from build123d import *

# Parameters (mm, degrees)
SKETCH1_R           = 2
SKETCH1_R_2         = 2.25
SKETCH1_R_3         = 16
SKETCH1_R_4         = 5.5
SKETCH1_R_5         = 1.75
SKETCH1_R_6         = 8.75
BOSS_EXTRUDE1_DEPTH = 3
SKETCH2_R           = 1.5
CUT_EXTRUDE1_DEPTH  = 190.515777006


with BuildPart() as part:
    # Sketch1 → Boss-Extrude1 (new body)
    with BuildSketch(Plane.XY):
        with BuildLine():
            ThreePointArc((-111.886028634, 49.480245878), (-128.824449864, 42.592956949), (-134.705774542, 25.279526249))
            ThreePointArc((-134.705774542, 25.279526249), (-136.343375771, 16.802270376), (-142.382746132, 10.632050724))
            ThreePointArc((-142.382746132, 10.632050724), (-155.099864059, -8.058287742), (-147.542861296, -29.364285714))
            ThreePointArc((-147.542861296, -29.364285714), (-143.125485566, -32.280163581), (-137.970351553, -33.480224156))
            ThreePointArc((-137.970351553, -33.480224156), (-126.431132561, -39.888203569), (-124.422839539, -52.93360637))
            ThreePointArc((-124.422839539, -52.93360637), (-124.888175134, -64.31939994), (-119.594822483, -74.410646153))
            Line((-119.594822483, -74.410646153), (-92.540517723, -103.740413224))
            ThreePointArc((-92.540517723, -103.740413224), (-82.119700521, -108.557935129), (-71.344567605, -104.595807028))
            Line((-71.344567605, -104.595807028), (-31.441449774, -67.788453323))
            ThreePointArc((-31.441449774, -67.788453323), (-26.802171393, -64.493076397), (-21.481893225, -62.473904985))
            Line((-21.481893225, -62.473904985), (87.599861039, -36.324111832))
            ThreePointArc((87.599861039, -36.324111832), (89.628937626, -35.308169791), (91, -33.5))
            ThreePointArc((91, -33.5), (97.203558128, 3.661751943), (84.51565505, 39.137054004))
            ThreePointArc((84.51565505, 39.137054004), (82.813644384, 40.69192784), (80.594954641, 41.317938046))
            Line((80.594954641, 41.317938046), (-111.886028634, 49.480245878))
        make_face()
        with Locations((-81.514845762, -93.570135067)):
            Circle(SKETCH1_R, mode=Mode.SUBTRACT)
        with Locations((-138.3, -22.75)):
            Circle(SKETCH1_R, mode=Mode.SUBTRACT)
        with Locations((-138.3, -5.25)):
            Circle(SKETCH1_R, mode=Mode.SUBTRACT)
        with Locations((-68.3, -21.5)):
            Circle(SKETCH1_R_2, mode=Mode.SUBTRACT)
        with Locations((-74.1, 1.7)):
            Circle(SKETCH1_R_2, mode=Mode.SUBTRACT)
        with Locations((-112.818118288, 27.5)):
            Circle(SKETCH1_R_3, mode=Mode.SUBTRACT)
        with Locations((-65.4, 20.2)):
            Circle(SKETCH1_R_2, mode=Mode.SUBTRACT)
        with Locations((18.5, -8.7)):
            Circle(SKETCH1_R_2, mode=Mode.SUBTRACT)
        with Locations((8.1, 8.2)):
            Circle(SKETCH1_R_2, mode=Mode.SUBTRACT)
        with Locations((75.9, -21.8)):
            Circle(SKETCH1_R_2, mode=Mode.SUBTRACT)
        with Locations((40.017782272, 0)):
            Circle(SKETCH1_R_4, mode=Mode.SUBTRACT)
        with Locations((78, -0.1)):
            Circle(SKETCH1_R_2, mode=Mode.SUBTRACT)
        with Locations((73, 22.4)):
            Circle(SKETCH1_R_2, mode=Mode.SUBTRACT)
        with Locations((-90.498978695, -58.098516388)):
            Circle(SKETCH1_R_5, mode=Mode.SUBTRACT)
        with Locations((-102.02811514, -72.419096433)):
            Circle(SKETCH1_R_5, mode=Mode.SUBTRACT)
        with Locations((-116.348695186, -60.889959988)):
            Circle(SKETCH1_R_5, mode=Mode.SUBTRACT)
        with Locations((-103.42383694, -59.494238188)):
            Circle(SKETCH1_R_6, mode=Mode.SUBTRACT)
        with Locations((-104.819558741, -46.569379943)):
            Circle(SKETCH1_R_5, mode=Mode.SUBTRACT)
    extrude(amount=BOSS_EXTRUDE1_DEPTH)

    # Sketch2 → Cut-Extrude1 (cut, through all)
    with BuildSketch(Plane.XY.offset(3)):
        with Locations((80.467851506, 38.32063179)):
            Circle(SKETCH2_R)
        with Locations((0.467851506, 41.713094856)):
            Circle(SKETCH2_R)
        with Locations((-79.532148494, 45.105557921)):
            Circle(SKETCH2_R)
        with Locations((86.900496491, -33.406768995)):
            Circle(SKETCH2_R)
        with Locations((9.034770729, -52.073251177)):
            Circle(SKETCH2_R)
        with Locations((-152.133709173, -14)):
            Circle(SKETCH2_R)
        with Locations((-68.830955034, -70.73973336)):
            Circle(SKETCH2_R)
    extrude(amount=-CUT_EXTRUDE1_DEPTH, mode=Mode.SUBTRACT)


solid = part.part
Could you check a few things on this model? Use its own coordinates, in mm. Round coordinates to 2 decimals unless told otherwise and drop trailing zeros. Order: outer loops, then holes, each group sorted by start corner. A loop starts at its lowest first (then second) coordinate and runs counter-clockwise, first axis right, second up.
Q1. Imagine slicing it at A-A, the plane z = 0.7. State how many separate pieces and enclosed holes the cut face has, then the cut area to 3 significant figures.
Geometry says:
separate pieces: 1
enclosed holes: 25
area: 24,800 mm2
Q2. Imagine slicing it at B-B, the plane x = -14. List the corners of the cut face in (y, z) for me, then the cut area to 3 significant figures.
Geometry says:
outline: (-60.68, 0) - (45.33, 0) - (45.33, 3) - (-60.68, 3) - close
area: 318 mm2
Q3. I'm going to push flat-ended pins straight in: P1, Ø5, axis at x = 80.47, y = 38.32, coming from the -Z side; P2, Ø1.5, axis at y = 19, z = 1, coming from the +X side; P3, Ø1.5, axis at y = -25, z = 1, coming from the -X side; P4, Ø1.5, axis at y = -31, z = 2, coming from the +X side. Where does each tip first touch, or does it pass through?
Geometry says:
P1: stops at z = 0
P2: stops at x = 94.42
P3: stops at x = -151.66
P4: stops at x = 92.36
Q4. Thinking about a two-plate mould opening in Y: for faces 1 (the face through (-128.803, 28.203, 1.479)), 2 (the face through (32.3, -49.58, 1.48)), 3 (the face through (97.25, 3.13, 1.48)), which applies, released by +Y, released by -Y, zero draft, split by the parting line, or undercut?
Geometry says:
face 1: undercut
face 2: released by -Y
face 3: split by the parting line
Q5. Imagine slicing it at C-C, the plane x = -42. List the corners of the cut face in (y, z) for me.
Geometry says:
outline: (-77.53, 0) - (46.52, 0) - (46.52, 3) - (-77.53, 3) - close
Q6. Please list where these lines run through material, in increasing order: probe 1 along Y at (x, z) = (-68, 0.55); probe 2 along X at (y, z) = (1.5, 2.75); probe 3 along X at (y, z) = (38.5, 1).
Geometry says:
probe 1: y = -101.51 to -71.99, -69.49 to -23.73, -19.27 to 47.62
probe 2: x = -151.81 to -76.34, -71.86 to 34.73, 45.31 to 76.42, 79.58 to 97.37
probe 3: x = -131.87 to -124.44, -101.2 to 78.98, 81.96 to 84.94
